Autodesk Inventor part; units mm, degrees
ref_plane "YZ Plane" through (0, 0, 0) normal (1, 0, 0) x (0, 1, 0)
ref_plane "XY Plane" through (0, 0, 0) normal (0, 0, 1) x (1, 0, 0)
sketch "Skizze1" plane through (0, 0, 0) normal (0, 0, 1) x (1, 0, 0)
  circle A0 centre (0, 0) radius 13
  line L0 (-18.2, 0) -> (18.2, 0)
  line L1 (0, -18.2) -> (0, 18.2)
  point P0 (0, 13)
  point P1 (0, -13)
  dimension "d0" = 26
revolve "Umdrehung1" add sketch "Skizze1" angle 360 about axis through (0, -10, 0) along (0, 1, 0) picked at (4.582, 7.2921) picked at (8.558, -0.9643) contours L0 L1 A0 | A0 L1 L0
sketch "Skizze2" plane through (0, 0, 0) normal (0, 0, 1) x (1, 0, 0)
  circle A0 centre (0, 0) radius 7.5
  dimension "d2" = 15
extrude "Extrusion1" cut sketch "Skizze2" along normal mid plane 26
ref_plane "Arbeitsebene1" through (0, 13, 0) normal (0, 1, 0) x (-1, 0, 0)
sketch "Skizze3" plane through (0, 13, 0) normal (0, 1, 0) x (-1, 0, 0)
  circle A0 centre (0, 0) radius 5
  dimension "d6" = 10
extrude "Extrusion2" add sketch "Skizze3" along normal blind 5 and the other way blind 1
sketch "Skizze4" plane through (0, 18, 0) normal (0, 1, 0) x (1, 0, 0)
  circle A0 centre (0, 0) radius 17
  dimension "d11" = 34
extrude "Extrusion3" add sketch "Skizze4" along normal blind 1
sketch "Skizze5" plane through (0, 19, 0) normal (0, 1, 0) x (1, 0, 0)
  circle A0 centre (0, 0) radius 17
  line L0 (5, 15.9474) -> (5, -15.9474)
  line L1 (7.5, 10.6184) -> (7.5, -10.6184)
  line L2 (5, 15.9474) -> (5, 16.2481)
  line L3 (5, -15.9474) -> (5, -16.2481)
  line L4 (-5, 16.2481) -> (-5, -16.2481)
  arc A1 (-5, -16.2481) -> (5, -16.2481) centre (0, 0) ccw
  arc A2 (5, 16.2481) -> (-5, 16.2481) centre (0, 0) ccw
  dimension "d15" = 5
  dimension "d16" = 5
extrude "Extrusion4" add sketch "Skizze5" along normal blind 3 contours L2 L0 L3 A0 L4
sketch "Skizze6" plane through (0, 22, 0) normal (0, 1, 0) x (1, 0, 0)
  line L0 (-5, 25) -> (5, 25)
  line L1 (5, 25) -> (5, -25)
  line L2 (5, -25) -> (-5, -25)
  line L3 (-5, -25) -> (-5, 25)
  line L4 (5, -16.2481) -> (5, 16.2481)
  point P0 (0, 0)
  dimension "d19" = 10
  dimension "d20" = 50
  dimension "d21" = 0
  dimension "d22" = 25
extrude "Extrusion5" add sketch "Skizze6" along normal blind 5
fillet "Rundung1" radius 2 18 edges at (0, 27, 25) (0, 22, 25) (5, 24.5, 25) (-5, 24.5, 25) (5, 27, 0) (-5, 27, 0) (5, 22, 20.624) (5, 20.5, 16.2481) (5, 22, -20.624) (5, 20.5, -16.2481) (-5, 22, 20.624) (-5, 20.5, 16.2481) (-5, 20.5, -16.2481) (-5, 22, -20.624) (-5, 24.5, -25) (0, 27, -25) (0, 22, -25) (5, 24.5, -25)
sketch "Skizze7" plane through (0, 27, 0) normal (0, 1, 0) x (1, 0, 0)
  circle A0 centre (0, 0) radius 3
  dimension "d26" = 6
extrude "Extrusion6" add sketch "Skizze7" along normal blind 15
properties part number "Ventilregler"
Could you check a few things on this model? Use its own coordinates, in mm. A direction names the side the tool comes from. Give positions to 0.01 mm unless a question says otherwise; leave off trailing zeros. Write each loop counter-clockwise with the first axis right and the second up, starting at its lowest first coordinate (ties: lowest second). Pieces come first, ordered by that corner, then holes. Notation, with made-up numbers: (27, 1) - (38, 1) arc R32 ccw to (38, 31) - close; hole circle Ø2 at (-16, -2.75). An arc over 180 degrees is marked (long way). One line per item, written item: value. Start each with the question number.
Item 1: Please list where these lines run through material, in increasing order: line 1 (Y direction, x = 0, z = 0.5); line 2 (Y direction, x = 0, z = 6.25); line 3 (X direction, y = 0, z = -0.25). Write a range as from..to.
Item 2: I'm going to push flat-ended pins straight in: pin 1 (8 mm diameter, centred on x = 7, z = -17, fed in from -Y); pin 2 (5 mm diameter, centred on x = -0.5, z = -20, fed in from -Y); pin 3 (6.5 mm diameter, centred on x = 0.5, z = -16, fed in from +Y); pin 4 (5 mm diameter, centred on x = 2, y = 22, fed in from +Z). Where does each tip first touch, or does it pass through?
Item 3: Imagine slicing it at B-B, the plane z = -21. List the corners of the cut face in (x, y) for me.
Item 4: Imagine slicing it at C-C, the plane y = 0. List the corners of the cut face in (x, z) for me, and give its area (3 significant figures).
Item 5: Imagine slicing it at D-D, the plane y = 16.5. List the corners of the cut face in (x, z) for me, and give its area (3 significant figures).
Item 6: Imagine slicing it at A-A, the plane x = 0. List the corners of the cut face in (y, z) for me, and give its area (3 significant figures).
Item 7: If we mould it in two halves opening along Y, with no side actions, what happens to faces 4 (the face through (-4.537, 20.979, -15.977)), 5 (the face through (4.43, 24.51, -24.4)), 6 (the face through (0, 22, 20))? For each: +Y half, -Y half, draft (parallel to the pull), parting line (faces both ways), or undercut.
Item 8: Which directions (+Z, -Z, +X, -X, +Y, -Y) give clear straight access to the entire face, cutting with the end or side of a thin tool? Please do faces 1 (the face through (1.08, 15.04, -4.88)), 2 (the face through (-17, 18.8, 0.2)), 3 (the face through (-3, 34, 0)).
Geometry says:
1. line 1: -12.99..-7.5, 7.5..42
1. line 2: -11.4..-7.5, 7.5..11.4, 18..27
1. line 3: -13..-7.5, 7.5..13
2. pin 1: y = 18
2. pin 2: y = 22
2. pin 3: y = 27
2. pin 4: z = 25
3. outline: (-5, 24) arc R2 ccw to (-3, 22) - (3, 22) arc R2 ccw to (5, 24) - (5, 25) arc R2 ccw to (3, 27) - (-3, 27) arc R2 ccw to (-5, 25) - close
4. outline: (-7.5, -10.62) - (-7.5, 10.62) arc R13 ccw to start; (7.5, -10.62) arc R13 ccw to (7.5, 10.62) - close
4. area: 164 mm^2
5. outline: circle Ø10 at (0, 0)
5. area: 78.5 mm^2
6. outline: (-7.5, -10.62) - (-7.5, 10.62) arc R13 ccw to start; (7.5, -10.62) arc R13 ccw to (12, -5) - (18, -5) - (18, -17) - (22, -17) - (22, -23) arc R2 ccw to (24, -25) - (25, -25) arc R2 ccw to (27, -23) - (27, -3) - (42, -3) - (42, 3) - (27, 3) - (27, 23) arc R2 ccw to (25, 25) - (24, 25) arc R2 ccw to (22, 23) - (22, 17) - (18, 17) - (18, 5) - (12, 5) arc R13 ccw to (7.5, 10.62) - close
6. area: 690 mm^2
7. face 4: undercut
7. face 5: draft
7. face 6: -Y half
8. face 1: none
8. face 2: -Y
8. face 3: +Y
